from build123d import *

# Parameters (mm, degrees)
SKETCH_1_W          = 40
SKETCH_1_H          = 40.5
EXTRUDE_1_DEPTH     = 20
SKETCH_2_R          = 6
EXTRUDE_2_DEPTH     = 2
SKETCH_4_R          = 2.5
EXTRUDE_3_DEPTH     = 2.5
SKETCH_5_R          = 2.5
EXTRUDE_4_DEPTH     = 2.5
SKETCH_6_R          = 1
CUT_EXTRUDE_1_DEPTH = 2.5
SKETCH_7_R          = 1
CUT_EXTRUDE_2_DEPTH = 2.5


with BuildPart() as part:
    # 草图1 → 凸台-拉伸1 (new body)
    with BuildSketch(Plane.XY):
        with Locations((20, 20.25)):
            Rectangle(SKETCH_1_W, SKETCH_1_H)
    extrude(amount=EXTRUDE_1_DEPTH)

    # 草图2 → 凸台-拉伸2 (add)
    with BuildSketch(Plane(origin=(0, 40.5, 0), x_dir=(1, 0, 0), z_dir=(0, 1, 0))):
        with Locations((30.1, -10)):
            Circle(SKETCH_2_R)
    extrude_2 = extrude(amount=EXTRUDE_2_DEPTH)

    # 镜向1: 凸台-拉伸2 across plane
    add(extrude_2.mirror(Plane.ZX.offset(20.25)))

    # 草图4 → 凸台-拉伸3 (add)
    with BuildSketch(Plane(origin=(0, 42.5, 0), x_dir=(1, 0, 0), z_dir=(0, 1, 0))):
        with Locations((30.1, -10)):
            Circle(SKETCH_4_R)
    extrude(amount=EXTRUDE_3_DEPTH)

    # 草图5 → 凸台-拉伸4 (add)
    with BuildSketch(Plane.XZ.offset(2)):
        with Locations((30.1, 10)):
            Circle(SKETCH_5_R)
    extrude(amount=EXTRUDE_4_DEPTH)

    # 草图6 → 切除-拉伸1 (cut)
    with BuildSketch(Plane(origin=(0, 40.5, 0), x_dir=(1, 0, 0), z_dir=(0, 1, 0))):
        with Locations((9.98, -3)):
            Circle(SKETCH_6_R)
        with Locations((9.98, -17)):
            Circle(SKETCH_6_R)
        with Locations((2.98, -10)):
            Circle(SKETCH_6_R)
    extrude(amount=-CUT_EXTRUDE_1_DEPTH, mode=Mode.SUBTRACT)

    # 草图7 → 切除-拉伸2 (cut)
    with BuildSketch(Plane.XZ):
        with Locations((2.5, 17.5)):
            Circle(SKETCH_7_R)
        with Locations((17.5, 17.5)):
            Circle(SKETCH_7_R)
        with Locations((17.5, 2.5)):
            Circle(SKETCH_7_R)
        with Locations((2.5, 2.5)):
            Circle(SKETCH_7_R)
    extrude(amount=-CUT_EXTRUDE_2_DEPTH, mode=Mode.SUBTRACT)


solid = part.part
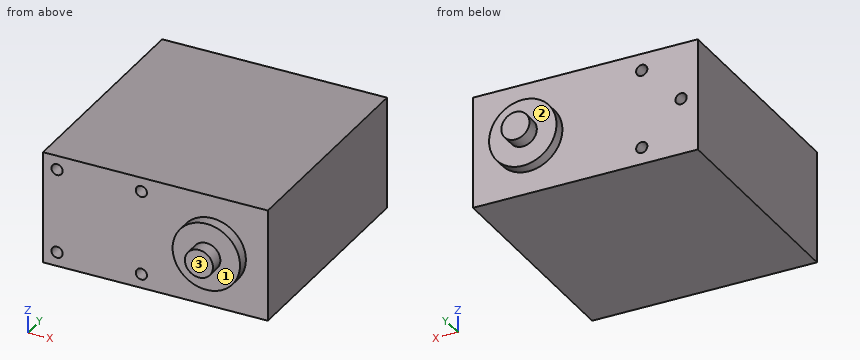
CAD build for the part. Positions are in the model's coordinates, mm. Face numbers are marked on the shaded views. A direction names the side the tool comes from. Give positions to 0.01 mm unless a question says otherwise; leave off trailing zeros. Order: outer loops, then holes, each group sorted by start corner. A loop starts at its lowest first (then second) coordinate and runs counter-clockwise, first axis right, second up. Notation, with made-up numbers: (78, -23.75) - (136, -23.75) arc R22 cw to (136, 11.25) - close; hole circle Ø9 at (-34, -5). An arc over 180 degrees is marked (long way). Write each question's results on one line, items separated by ' | '.
1. Saw through at C-C on x = 21.5. List the corners of the cut face in (y, z), and give its area (3 significant figures).
Calculated:
outline: (0, 0) - (40.5, 0) - (40.5, 20) - (0, 20) - close | area: 810 mm2
2. Saw through at B-B on x = 17.5. List the corners of the cut face in (y, z).
Calculated:
outline: (0, 0) - (40.5, 0) - (40.5, 20) - (0, 20) - (0, 18.5) - (2.5, 18.5) - (2.5, 16.5) - (0, 16.5) - (0, 3.5) - (2.5, 3.5) - (2.5, 1.5) - (0, 1.5) - close
3. Pin check, flat tips, straight feed: pin 1 (2.5 mm diameter, centred on x = 2.5, z = 2.5, fed in from +Y); pin 2 (1.6 mm diameter, centred on x = 17, z = 17.5, fed in from -Y); pin 3 (0.6 mm diameter, centred on x = 3.5, z = 10, fed in from +Y). Stop position of each tip, or through.
Calculated:
pin 1: stops at y = 40.5 | pin 2: stops at y = 0 | pin 3: stops at y = 38
4. 3-axis set-ups, long thin cutter, end or side, ignore diameter. For the marked faces 1, 2 and 3: which of +Z, -Z, +X, -X, +Y, -Y reach the whole face in a straight line?
Calculated:
face 1: -Y | face 2: +Y | face 3: +Z, -Z, +X, -X, -Y
5. Saw through at A-A on z = 10. List the corners of the cut face in (x, y), and give its area (3 significant figures).
Calculated:
outline: (0, 0) - (24.1, 0) - (24.1, -2) - (27.6, -2) - (27.6, -4.5) - (32.6, -4.5) - (32.6, -2) - (36.1, -2) - (36.1, 0) - (40, 0) - (40, 40.5) - (36.1, 40.5) - (36.1, 42.5) - (32.6, 42.5) - (32.6, 45) - (27.6, 45) - (27.6, 42.5) - (24.1, 42.5) - (24.1, 40.5) - (3.98, 40.5) - (3.98, 38) - (1.98, 38) - (1.98, 40.5) - (0, 40.5) - close | area: 1,690 mm2
6. Probe L1, parallel to Z at x = 9.98, y = 38.7; L2, parallel to Z at x = 2.5, y = 2.05; L3, parallel to X at y = 39.1, z = 17. List the from-to ranges inside material, lowest first. Write a range as from..to.
Calculated:
L1: z = 0..2, 4..16, 18..20 | L2: z = 0..1.5, 3.5..16.5, 18.5..20 | L3: x = 0..8.98, 10.98..40
